```python
from build123d import *

# Parameters (mm, degrees)
SKETCH_W      = 48
SKETCH_H      = 28
PAD_DEPTH     = 2
SKETCH001_R   = 1
PAD001_DEPTH  = 3
SKETCH003_W   = 1.5
SKETCH003_H   = 3
SKETCH003_W_2 = 3
SKETCH003_H_2 = 10.8
POCKET_DEPTH  = 5.001
SKETCH004_W   = 22
SKETCH004_H   = 1.5
PAD002_DEPTH  = 2.4


with BuildPart() as part:
    # Sketch → Pad (new body)
    with BuildSketch(Plane.XY):
        with Locations((24, 14)):
            Rectangle(SKETCH_W, SKETCH_H)
    extrude(amount=PAD_DEPTH)

    # Sketch001 → Pad001 (new body)
    with BuildSketch(Plane.XY.offset(2)):
        with Locations((2.2, 2.2)):
            Circle(SKETCH001_R)
        with Locations((2.2, 25.8)):
            Circle(SKETCH001_R)
        with Locations((45.8, 25.8)):
            Circle(SKETCH001_R)
        with Locations((45.8, 2.2)):
            Circle(SKETCH001_R)
    extrude(amount=PAD001_DEPTH)

    # Sketch003 → Pocket (cut, through all)
    with BuildSketch(Plane(origin=(0, 0, 0), x_dir=(1, 0, 0), z_dir=(0, 0, -1))):
        with Locations((5.25, -6.2)):
            Rectangle(SKETCH003_W, SKETCH003_H)
        with Locations((5.25, -23.82386)):
            Rectangle(SKETCH003_W, SKETCH003_H)
        with Locations((42.45, -23.82386)):
            Rectangle(SKETCH003_W, SKETCH003_H)
        with Locations((42.2, -14)):
            Rectangle(SKETCH003_W_2, SKETCH003_H_2)
    extrude(amount=-POCKET_DEPTH, mode=Mode.SUBTRACT)

    # Sketch004 → Pad002 (new body)
    with BuildSketch(Plane.XY.offset(2)):
        with Locations((20, 5.75)):
            Rectangle(SKETCH004_W, SKETCH004_H)
        with Locations((20, 23.526215)):
            Rectangle(SKETCH004_W, SKETCH004_H)
    extrude(amount=PAD002_DEPTH)


solid = part.part
```
Read the model definition and answer for the solid it produces. Units are mm, in the model's axes. A direction names the side the tool comes from. Coordinates: 2 decimals unless noted, no trailing zeros. Write each loop counter-clockwise with the first axis right and the second up, starting at its lowest first coordinate (ties: lowest second). Pieces come first, ordered by that corner, then holes. Notation, with made-up numbers: (65.25, 52) - (120.25, 52) arc R37 ccw to (120.25, 90) - close; hole circle Ø9 at (48, -40). An arc over 180 degrees is marked (long way). Answer as a JSON object with one key per item and string values. Group by question number.
1. Each of these flat-tipped pins is pushed along its axis until it touches: P1, Ø0.8, axis at y = 5.5, z = 3.5, coming from the +X side; P2, Ø2.5, axis at x = 18, z = 3.5, coming from the -Y side; P3, Ø2.5, axis at x = 25, z = 3.5, coming from the +Y side. Where does it stop, or does it pass through?
2. Which of the six approach directions +Z, -Z, +X, -X, +Y, -Y give full straight-line access (tool end or side, diameter ignored) to faces 5 (the flat face through (4.5, 6, 1)), 6 (the flat face through (46, 2, 5)), 7 (the flat face through (9, 6, 3)), 8 (the flat face through (24, 14, 2)), 9 (the flat face through (20, 24.276, 3))?
3. The mould has two halves that part along Y. Classify faces 1 (the cylindrical face through (45, 25.2, 3.5)), 2 (the flat face through (24, 28, 1)), 3 (the flat face through (20, 5, 3)), 4 (the flat face through (43.7, 14, 1)): +Y half, -Y half, draft (parallel to the pull), parting line (faces both ways), or undercut.
4. A cutting plane is placed at C-C (x = 21.5). Determine the outline of the cut face in (y, z).
5. A cutting plane is placed at D-D (y = 16). Determine the outline of the cut face in (x, z).
6. Consider L1, parallel to X at y = 23.75, z = 0.9; L2, parallel to X at y = 7.5, z = 0.6; L3, parallel to Y at x = 14.5, z = 2.4. Determine where each line is inside the solid, lowest interval first. Write a range as [from, to].
7. A cutting plane is placed at B-B (y = 23.25). Determine the outline of the cut face in (x, z), plus the area to 3 significant figures.
8. A cutting plane is placed at A-A (z = 3). Determine the outline of the cut face in (x, y).
Worked out:
{
 "1": {"P1": "stops at x = 31", "P2": "stops at y = 5", "P3": "stops at y = 24.28"},
 "2": {"face 5": "+Z, -Z", "face 6": "+Z, +X, -X, +Y, -Y", "face 7": "+Z, -X, +Y, -Y", "face 8": "+Z", "face 9": "+Z, +X, -X, +Y"},
 "3": {"face 1": "undercut", "face 2": "+Y half", "face 3": "-Y half", "face 4": "undercut"},
 "4": {"outline": "(0, 0) - (28, 0) - (28, 2) - (24.28, 2) - (24.28, 4.4) - (22.78, 4.4) - (22.78, 2) - (6.5, 2) - (6.5, 4.4) - (5, 4.4) - (5, 2) - (0, 2) - close"},
 "5": {"outline": "(0, 0) - (40.7, 0) - (40.7, 2) - (0, 2) - close; (43.7, 0) - (48, 0) - (48, 2) - (43.7, 2) - close"},
 "6": {"L1": "x = [0, 4.5], [6, 41.7], [43.2, 48]", "L2": "x = [0, 4.5], [6, 48]", "L3": "y = [5, 6.5], [22.78, 24.28]"},
 "7": {"outline": "(0, 0) - (4.5, 0) - (4.5, 2) - (0, 2) - close; (6, 0) - (41.7, 0) - (41.7, 2) - (31, 2) - (31, 4.4) - (9, 4.4) - (9, 2) - (6, 2) - close; (43.2, 0) - (48, 0) - (48, 2) - (43.2, 2) - close", "area": "143 mm²"},
 "8": {"outline": "circle Ø2 at (2.2, 2.2); circle Ø2 at (2.2, 25.8); (9, 5) - (31, 5) - (31, 6.5) - (9, 6.5) - close; (9, 22.78) - (31, 22.78) - (31, 24.28) - (9, 24.28) - close; circle Ø2 at (45.8, 2.2); circle Ø2 at (45.8, 25.8)"}
}
